```python
from build123d import *

# Parameters (mm, degrees)
F0_W     = 76.2
F0_H     = 101.6
F1_DEPTH = 9.525
F2_SIZE  = 9.52499
F3_R     = 15.875
F4_DEPTH = 9.525


# Not quite as in the source:
# - a fillet or chamfer is up to 0.001 mm smaller than in the source, because OpenCascade refuses the exact size


with BuildPart() as f1:
    # F0 (on Top) → F1 (new body)
    with BuildSketch(Plane.XY):
        Rectangle(F0_W, F0_H)
    extrude(amount=F1_DEPTH)

    # F2 (size 9.525 in the source; OpenCascade refuses exactly that, so slightly less here)
    f2_edges = [f1.edges().sort_by_distance(p)[0] for p in [
        (0, -50.8, 9.525),
    ]]
    chamfer(f2_edges, length=F2_SIZE)

    # F3 (on face) → F4 (cut)
    with BuildSketch(Plane(origin=(0, 0, 0), x_dir=(1, 0, 0), z_dir=(0, 0, -1))):
        with Locations((0, -25.4)):
            Circle(F3_R)
    extrude(amount=-F4_DEPTH, mode=Mode.SUBTRACT)


solid = f1.part
```
Geometry check sheet. Reference: the model listing, model coordinates, mm. Round coordinates to 2 decimals unless told otherwise and drop trailing zeros. Loops run counter-clockwise (first coordinate to the right, second up) from the corner with the lowest first, then second, coordinate; pieces in that order, holes last. Notation, with made-up numbers: (60, 40) - (108, 40) arc R30 cw to (108, 64) - close; hole circle Ø6 at (15, 37.5). An arc over 180 degrees is marked (long way). Write each question's results on one line, items separated by ' | '. Start each with the question number.
Q1. Cross-section at D-D on z = 4. Enter the section's corners in (x, y) (3 decimals), and give its area (3 significant figures).
Q2. Cross-section at A-A on y = 25.4. Enter the section's corners in (x, z) (3 decimals).
Q3. Gauge pin test, flat end, axial feed: P1, Ø4, axis at x = -11, y = 40.5, coming from the -Z side. Record the tip position at first contact, or that the pin passes through.
Q4. Release check for a two-part mould opening along Y. For faces 1 (the flat face through (-1, 50.8, 5)), 2 (the flat face through (38.1, -1, 5)), 3 (the flat face through (-0.5, -46, 4.8)), 4 (the cylindrical face through (-2.07, 9.66, 4.7)) record: +Y half, -Y half, draft (parallel to the pull), parting line (faces both ways), or undercut.
Q5. Thickness scan on line 1 (X direction, y = 25.4, z = 2) (3 decimals); line 2 (X direction, y = 24.5, z = 7.75); line 3 (Y direction, x = 0, z = 4) (3 decimals). Record the ranges inside material, lowest first. Write a range as [from, to].
Answers below:
1) outline: (-38.1, -46.8) - (38.1, -46.8) - (38.1, 50.8) - (-38.1, 50.8) - close; hole circle Ø31.75 at (0, 25.4) | area: 6,650 mm²
2) outline: (-38.1, 0) - (-15.875, 0) - (-15.875, 9.525) - (-38.1, 9.525) - close; (15.875, 0) - (38.1, 0) - (38.1, 9.525) - (15.875, 9.525) - close
3) P1: stops at z = 0
4) face 1: +Y half | face 2: draft | face 3: -Y half | face 4: undercut
5) line 1: x = [-38.1, -15.875], [15.875, 38.1] | line 2: x = [-38.1, -15.85], [15.85, 38.1] | line 3: y = [-46.8, 9.525], [41.275, 50.8]
